Autodesk Inventor part; units mm, degrees
ref_plane "YZ Plane" through (0, 0, 0) normal (1, 0, 0) x (0, 1, 0)
ref_plane "XZ Plane" through (0, 0, 0) normal (0, 1, 0) x (-1, 0, 0)
ref_plane "XY Plane" through (0, 0, 0) normal (0, 0, 1) x (1, 0, 0)
sketch "Sketch1" plane through (0, 0, 0) normal (0, 0, 1) x (1, 0, 0)
  line L0 (0, -5) -> (0, 5) construction
  line L1 (1, -5) -> (1, 5)
  line L2 (-1, 5) -> (-1, -5)
  arc A0 (-1, -5) -> (1, -5) centre (0, -5) ccw
  arc A1 (1, 5) -> (-1, 5) centre (0, 5) ccw
  line L3 (0, -6) -> (0, 6) construction
  line L4 (-4, -6) -> (-4, 6)
  line L5 (4, 6) -> (4, -6)
  arc A2 (-4, -6) -> (4, -6) centre (0, -6) ccw
  arc A3 (4, 6) -> (-4, 6) centre (0, 6) ccw
  point P0 (0, 0)
  dimension "d0" = 5
  dimension "d1" = 2
  dimension "d2" = 1
  dimension "d3" = 3
extrude "Extrusion1" add sketch "Sketch1" along normal blind 6.5
properties part number "COILS" material "Copper"
Can you work these out from the model? Positions are in its coordinate system, mm. A direction names the side the tool comes from. Coordinates: 2 decimals unless noted, no trailing zeros. Order: outer loops, then holes, each group sorted by start corner. A loop starts at its lowest first (then second) coordinate and runs counter-clockwise, first axis right, second up. Notation, with made-up numbers: M 33.5,2.25 L 68.5,2.25 A25 cw 68.5,29.25 Z; hole C 1.5,68.25 d8. An arc over 180 degrees is marked long. Answer as CSV lines item,"result".
(1) I'm going to push flat-ended pins straight in: pin 1 (1 mm diameter, centred on x = 3, z = 4.5, fed in from -Y); pin 2 (1 mm diameter, centred on x = -0.5, z = 1.5, fed in from +Y); pin 3 (3 mm diameter, centred on x = -2.5, z = 2.5, fed in from -Y); pin 4 (2 mm diameter, centred on x = -2.5, z = 4.5, fed in from -Y). Where does each tip first touch, or does it pass through?
Geometry check:
pin 1,"y = -9.12"
pin 2,"y = 10"
pin 3,"y = -9.87"
pin 4,"y = -9.71"
(2) On a 3-axis mill with a long thin cutter (end or side, diameter ignored), from which of +Z, -Z, +X, -X, +Y, -Y can I reach the whole of each face in a straight line? I mean faces 4 (the cylindrical face through (0, 6, 3)), 5 (the cylindrical face through (0, -10, 3)). Say none if no direction works.
Geometry check:
face 4,"+Z, -Z"
face 5,"+Z, -Z, -Y"
(3) Suppose I cut it at A-A on x = 0. Please give me the cut outline in (y, z).
Geometry check:
outline,"M -10,0 L -6,0 L -6,6.5 L -10,6.5 Z; M 6,0 L 10,0 L 10,6.5 L 6,6.5 Z"
(4) Suppose I cut it at B-B on y = 2.5. Please give me the cut outline in (x, z), plus the area to 3 significant figures.
Geometry check:
outline,"M -4,0 L -1,0 L -1,6.5 L -4,6.5 Z; M 1,0 L 4,0 L 4,6.5 L 1,6.5 Z"
area,"39.0 mm^2"
(5) Suppose I cut it at D-D on x = -3. Please give me the cut outline in (y, z).
Geometry check:
outline,"M -8.65,0 L 8.65,0 L 8.65,6.5 L -8.65,6.5 Z"
(6) If we mould it in two halves opening along X, with no side actions, what happens to faces 1 (the flat face through (4, 0, 3)), 2 (the flat face through (2, 0, 6.5)), 3 (the cylindrical face through (0, -6, 3))? For each: released by +X, released by -X, zero draft, split by the parting line, or undercut.
Geometry check:
face 1,"released by +X"
face 2,"zero draft"
face 3,"undercut"
(7) Please list where these lines run through material, in increasing order: L1, parallel to X at y = -4.25, z = 0.75; L2, parallel to X at y = 5.5, z = 5.5; L3, parallel to Y at x = -3.5, z = 2.25.
Geometry check:
L1,"-4 to -1, 1 to 4"
L2,"-4 to -0.87, 0.87 to 4"
L3,"-7.94 to 7.94"
(8) Suppose I cut it at C-C on z = 2.75. Please give me the cut outline in (x, y).
Geometry check:
outline,"M -4,-6 A4 ccw 4,-6 L 4,6 A4 ccw -4,6 Z; hole M -1,-5 A1 ccw 1,-5 L 1,5 A1 ccw -1,5 Z"
